```python
from build123d import *

# Parameters (mm, degrees)
EXTRUDE_2_OUTLINE_R   = 3
EXTRUDE_2_OUTLINE_R_2 = 2.1
EXTRUDE_2_DEPTH       = 5
FILLET_1_R            = 5
CHAMFER_1_SIZE        = 1
CHAMFER_2_SIZE        = 1


# Read off the part's stored shape, not the designer's step: ﾎﾞｽ - 押し出し2
with BuildPart() as part:
    # ﾎﾞｽ - 押し出し2 outline → ﾎﾞｽ - 押し出し2 (new body)
    with BuildSketch(Plane(origin=(0, 0, 0), x_dir=(1, 0, 0), z_dir=(0, 1, 0))):
        with BuildLine():
            Line((-25.627313747, -23.456190528), (-13.58012702, -16.500744028))
            Line((-13.58012702, -16.500744028), (-4.330127019, -32.522214))
            ThreePointArc((-4.330127019, -32.522214), (0, -35.022214), (4.330127019, -32.522214))
            Line((4.330127019, -32.522214), (13.595203608, -16.474630613))
            Line((13.595203608, -16.474630613), (25.627663459, -23.456392422))
            ThreePointArc((25.627663459, -23.456392422), (35.872706169, -20.710650288), (33.126964036, -10.465607578))
            Line((33.126964036, -10.465607578), (21.079752539, -3.511011592))
            Line((21.079752539, -3.511011592), (30.330127021, 12.511107))
            ThreePointArc((30.330127021, 12.511107), (30.330127021, 17.511107), (26.000000002, 20.011107))
            Line((26.000000002, 20.011107), (7.500451194, 20.011107))
            Line((7.500451194, 20.011107), (7.500451194, 33.922))
            ThreePointArc((7.500451194, 33.922), (0, 41.422451194), (-7.500451194, 33.922))
            Line((-7.500451194, 33.922), (-7.500451194, 20.011107))
            Line((-7.500451194, 20.011107), (-26.000000002, 20.011107))
            ThreePointArc((-26.000000002, 20.011107), (-30.330127021, 17.511107), (-30.330127021, 12.511107))
            Line((-30.330127021, 12.511107), (-21.08012702, -3.510362972))
            Line((-21.08012702, -3.510362972), (-33.127313747, -10.465809472))
            ThreePointArc((-33.127313747, -10.465809472), (-35.872504276, -20.711), (-25.627313747, -23.456190528))
        make_face()
        with Locations((-29.377313747, -16.961)):
            Circle(EXTRUDE_2_OUTLINE_R, mode=Mode.SUBTRACT)
        with Locations((0, -30.022214)):
            Circle(EXTRUDE_2_OUTLINE_R_2, mode=Mode.SUBTRACT)
        with Locations((29.377313747, -16.961)):
            Circle(EXTRUDE_2_OUTLINE_R, mode=Mode.SUBTRACT)
        with Locations((-26.000000002, 15.011107)):
            Circle(EXTRUDE_2_OUTLINE_R_2, mode=Mode.SUBTRACT)
        with Locations((26.000000002, 15.011107)):
            Circle(EXTRUDE_2_OUTLINE_R_2, mode=Mode.SUBTRACT)
        with Locations((0, 33.922)):
            Circle(EXTRUDE_2_OUTLINE_R, mode=Mode.SUBTRACT)
    extrude(amount=EXTRUDE_2_DEPTH)

    # ﾌｨﾚｯﾄ1
    fillet_1_edges = [part.edges().sort_by_distance(p)[0] for p in [
        (-13.58012702, 2.5, 16.500744028),
        (-21.08012702, 2.5, 3.510362972),
        (-7.500451194, 2.5, -20.011107),
        (7.500451194, 2.5, -20.011107),
        (21.079752539, 2.5, 3.511011592),
        (13.595203608, 2.5, 16.474630613),
    ]]
    fillet(fillet_1_edges, radius=FILLET_1_R)

    # 面取り1
    chamfer_1_edges = [part.edges().sort_by_distance(p)[0] for p in [
        (-14.116158813, 0, 18.501241916),
        (-21.768783893, 0, 21.228467278),
        (-35.872504276, 0, 20.711),
        (-29.268783893, 0, 8.238086222),
        (-30.330127021, 0, -17.511107),
        (-19.250225598, 0, -20.011107),
        (-7.500451194, 0, -29.4665535),
        (0, 0, -41.422451194),
        (7.500451194, 0, -29.4665535),
        (30.330127021, 0, -17.511107),
        (26.955007083, 0, -6.665227785),
        (29.26860567, 0, 8.238260311),
        (35.872706169, 0, 20.710650288),
        (21.778474587, 0, 21.222923938),
        (0, 0, 35.022214),
        (-7.705127019, 0, 26.676542524),
        (7.709952964, 0, 26.668183744),
        (19.250225598, 0, -20.011107),
        (-26.95512702, 0, -6.665435523),
        (14.131045637, 0, 18.483124699),
        (23.080419871, 0, 2.97487667),
        (8.964917288, 0, -21.475573094),
        (-8.964917288, 0, -21.475573094),
        (-23.080624907, 0, 2.974331179),
    ]]
    chamfer(chamfer_1_edges, length=CHAMFER_1_SIZE)

    # 面取り2
    chamfer_2_edges = [part.edges().sort_by_distance(p)[0] for p in [
        (-7.705127019, 5, 26.676542524),
        (-23.080624907, 5, 2.974331179),
        (-14.116158813, 5, 18.501241916),
        (0, 5, 35.022214),
        (21.778474587, 5, 21.222923938),
        (35.872706169, 5, 20.710650288),
        (29.26860567, 5, 8.238260311),
        (26.955007083, 5, -6.665227785),
        (30.330127021, 5, -17.511107),
        (7.500451194, 5, -29.4665535),
        (0, 5, -41.422451194),
        (-7.500451194, 5, -29.4665535),
        (-19.250225598, 5, -20.011107),
        (-30.330127021, 5, -17.511107),
        (-29.268783893, 5, 8.238086222),
        (-35.872504276, 5, 20.711),
        (7.709952964, 5, 26.668183744),
        (-21.768783893, 5, 21.228467278),
        (19.250225598, 5, -20.011107),
        (-26.95512702, 5, -6.665435523),
        (14.131045637, 5, 18.483124699),
        (23.080419871, 5, 2.97487667),
        (8.964917288, 5, -21.475573094),
        (-8.964917288, 5, -21.475573094),
    ]]
    chamfer(chamfer_2_edges, length=CHAMFER_2_SIZE)


solid = part.part
```
The model under review builds one solid part; all positions refer to its coordinate system, in mm. A direction names the side the tool comes from. Round coordinates to 2 decimals unless told otherwise and drop trailing zeros. Order: outer loops, then holes, each group sorted by start corner. A loop starts at its lowest first (then second) coordinate and runs counter-clockwise, first axis right, second up. Notation, with made-up numbers: (24.5, -12) -> (63.5, -12) arc R24 cw to (63.5, 16) -> close; hole circle Ø2 at (74.5, 47). An arc over 180 degrees is marked (long way). Use a Markdown table: item, result.
Q1. For line 1 (Z direction, x = 0.5, y = 4.2); line 2 (X direction, y = 0.55, z = -13.5); line 3 (X direction, y = 0.5, z = 31.5), list the stretches that pass through material, from the lowest coordinate up.
Values:
| item | result |
|---|---|
| line 1 | z = -41.21 to -36.88, -30.96 to 27.98, 32.06 to 34.8 |
| line 2 | x = -30.29 to -27.46, -24.54 to 24.54, 27.46 to 30.29 |
| line 3 | x = -4.34 to -1.49, 1.49 to 4.34 |
Q2. We need section C-C on z = -6. Write out the cut boundary in (x, y).
Values:
| item | result |
|---|---|
| outline | (-26.57, 1) -> (-25.42, 0) -> (25.42, 0) -> (26.57, 1) -> (26.57, 4) -> (25.42, 5) -> (-25.42, 5) -> (-26.57, 4) -> close |
Q3. Tool access review of faces 1 (the flat face through (-27.002, 2.479, -6.747)), 2 (the flat face through (-21.82, 2.48, 21.26)), 3 (the flat face through (26.481, 0.507, -6.83)): name each direction out of +Z, -Z, +X, -X, +Y, -Y from which nothing blocks a thin tool from reaching the whole face with its end or side.
Values:
| item | result |
|---|---|
| face 1 | -X, +Y, -Y |
| face 2 | +Z, +Y, -Y |
| face 3 | +X, -Y |
Q4. Mouldability with a two-part tool opening along X and no side actions: class faces 4 (the cylindrical face through (23.095, 2.521, 3.028)), 5 (the flat face through (-7.33, 4.49, 26.35)), 6 (the flat face through (-28.97, 4.49, 8.63)) as +X half, -X half, draft (parallel to the pull), parting line (faces both ways), or undercut.
Values:
| item | result |
|---|---|
| face 4 | +X half |
| face 5 | undercut |
| face 6 | -X half |
Q5. We need section D-D on z = 9.5. Write out the cut boundary in (x, y).
Values:
| item | result |
|---|---|
| outline | (-31.45, 1) -> (-29.45, 0) -> (29.45, 0) -> (31.45, 1) -> (31.45, 4) -> (29.45, 5) -> (-29.45, 5) -> (-31.45, 4) -> close |
Q6. We need section A-A on x = 0. Write out the cut boundary in (y, z).
Values:
| item | result |
|---|---|
| outline | (0, -40.42) -> (1, -41.42) -> (4, -41.42) -> (5, -40.42) -> (5, -36.92) -> (0, -36.92) -> close; (0, -30.92) -> (5, -30.92) -> (5, 27.92) -> (0, 27.92) -> close; (0, 32.12) -> (5, 32.12) -> (5, 34.02) -> (4, 35.02) -> (1, 35.02) -> (0, 34.02) -> close |
Q7. Clearance check with flat-ended pins moving along their axes: P1, Ø3, axis at x = -20.5, y = 1.5, coming from the -Z side; P2, Ø2, axis at y = 1, z = -17, coming from the +X side; P3, Ø2, axis at y = 0.5, z = -22.5, coming from the +X side. State where each tip first meets the part, or that it passes through.
Values:
| item | result |
|---|---|
| P1 | stops at z = -20.01 |
| P2 | stops at x = 30.9 |
| P3 | stops at x = 8.81 |
Q8. We need section B-B on y = 3.15. State how many separate pieces and enclosed holes the cut face has, then the cut area to 3 significant figures.
Values:
| item | result |
|---|---|
| separate pieces | 1 |
| enclosed holes | 6 |
| area | 2,830 mm^2 |
